For this review, take the finished solid that the model builds, in its own axes (mm). A direction names the side the tool comes from. Round coordinates to 2 decimals unless told otherwise and drop trailing zeros. Loops run counter-clockwise (first coordinate to the right, second up) from the corner with the lowest first, then second, coordinate; pieces in that order, holes last. Notation, with made-up numbers: (33, 61) -> (47, 61) arc R22 ccw to (47, 90) -> close; hole circle Ø1 at (54.25, 54.25). An arc over 180 degrees is marked (long way). Use one line per item in the form item = value. Start each with the question number.
from build123d import *

# Parameters (mm, degrees)
SWEEP1_PROFILE_R   = 15
SKETCH26_W         = 20
SKETCH26_H         = 24.358108154
CUT_EXTRUDE2_DEPTH = 237.5
CUT_EXTRUDE3_START = -950
SKETCH26_2_W       = 20
SKETCH26_2_H       = 24.358108154
CUT_EXTRUDE3_DEPTH = 237.5


with BuildPart() as part:
    # Sweep1: sweep along a path in Sketch1
    with BuildLine(Plane.XY) as sweep1_path:
        Line((-475, 0), (-257.280174441, 0))
        ThreePointArc((-257.280174441, 0), (-237.625861021, 1.110364069), (-218.221667938, 4.42732581))
        Line((-218.221667938, 4.42732581), (-39.058506504, 45.57267419))
        ThreePointArc((-39.058506504, 45.57267419), (0, 50), (39.058506504, 45.57267419))
        Line((39.058506504, 45.57267419), (218.221667938, 4.42732581))
        ThreePointArc((218.221667938, 4.42732581), (237.625861021, 1.110364069), (257.280174441, 0))
        Line((257.280174441, 0), (475, 0))
    # Sweep1 profile (on start of the path) → Sweep1 (sweep)
    with BuildSketch(Plane(origin=(-475, 0, 0), x_dir=(0, 0, 1), z_dir=(1, 0, 0))):
        Circle(SWEEP1_PROFILE_R)
    sweep(path=sweep1_path.line)

    # Sketch26 → Cut-Extrude2 (cut)
    with BuildSketch(Plane.ZY.offset(475)):
        with Locations((0, -15)):
            Rectangle(SKETCH26_W, SKETCH26_H)
    extrude(amount=-CUT_EXTRUDE2_DEPTH, mode=Mode.SUBTRACT)

    # Sketch26<2> → Cut-Extrude3 (cut)
    with BuildSketch(Plane.ZY.offset(475).offset(CUT_EXTRUDE3_START)):
        with Locations((0, -15)):
            Rectangle(SKETCH26_2_W, SKETCH26_2_H)
    extrude(amount=CUT_EXTRUDE3_DEPTH, mode=Mode.SUBTRACT)


solid = part.part
Item 1: Machinability: for faces 4 (the flat face through (-358, -2.821, 0)), 5 (the cylindrical face through (-364.62, 14.99, -0.51)), 6 (the cylindrical face through (367.66, 14.99, -0.51)), which of the approach directions +Z, -Z, +X, -X, +Y, -Y give a long, thin tool a straight path to every point of the face, cutting with its end or side? Answer none if there is none.
Item 2: For P1, Ø4, axis at x = -28, z = 10.5, coming from the +Y side; P2, Ø4, axis at x = 226.5, z = -6, coming from the +Y side; P3, Ø6.5, axis at x = 400, y = -8.5, coming from the -Z side; P4, Ø9, axis at y = -6, z = -1.5, coming from the +X side, all flat-tipped, find the tip position at first contact; note any pin that passes through.
Item 3: Draft analysis for pull direction Z (two halves, no side actions). For faces 1 (the flat face through (-475, 5, 0)), 2 (the cylindrical face through (131.94, 33.61, -11.9)), 3 (the flat face through (358, -2.821, 0)), state which applies: +Z half, -Z half, draft (parallel to the pull), parting line (faces both ways), or undercut.
Item 4: Wall thickness on line 1 (Z direction, x = -248, y = 0); line 2 (Z direction, x = 293, y = -3); line 3 (Z direction, x = -25.5, y = 58.5): over which ranges is each line inside the solid? List them lowest first.
Item 5: Take a section at A-A on z = 0. Give the boundary of the cut face in (x, y), plus the area to 3 significant figures.
Results:
q1.face_4 = -X, -Y
q1.face_5 = -X
q1.face_6 = +X
q2.P1 = 60.28
q2.P2 = 17.57
q2.P3 = -14.05
q2.P4 = 475
q3.face_1 = draft
q3.face_2 = parting line
q3.face_3 = undercut
q4.line_1 = -15 to 15
q4.line_2 = -14.7 to -10, 10 to 14.7
q4.line_3 = -10.93 to 10.93
q5.outline = (-475, -2.82) -> (-237.5, -2.82) -> (-237.5, -13.96) arc R189.5 ccw to (-214.86, -10.19) -> (-35.7, 30.95) arc R159.5 cw to (35.7, 30.95) -> (214.86, -10.19) arc R189.5 ccw to (237.5, -13.96) -> (237.5, -2.82) -> (475, -2.82) -> (475, 15) -> (257.28, 15) arc R159.5 cw to (221.58, 19.05) -> (42.42, 60.19) arc R189.5 ccw to (-42.42, 60.19) -> (-221.58, 19.05) arc R159.5 cw to (-257.28, 15) -> (-475, 15) -> close
q5.area = 23,000 mm2
